from build123d import *

# Parameters (mm, degrees)
F0_W     = 50.8
F0_H     = 31.75
F1_DEPTH = 31.75
F2_W     = 25.4
F2_H     = 19.05
F3_DEPTH = 31.751
F4_R     = 25.4
F5_DEPTH = 50.801


with BuildPart() as f1:
    # F0 (on Front) → F1 (new body)
    with BuildSketch(Plane.XZ):
        with Locations((25.4, 15.875)):
            Rectangle(F0_W, F0_H)
    extrude(amount=F1_DEPTH)

    # F2 (on face) → F3 (cut, through all)
    with BuildSketch(Plane.XZ.offset(31.75)):
        with Locations((25.4, 22.225)):
            Rectangle(F2_W, F2_H)
    extrude(amount=-F3_DEPTH, mode=Mode.SUBTRACT)

    # F4 (on face) → F5 (cut, through all)
    with BuildSketch(Plane.YZ.offset(50.8)):
        with Locations((-31.75, 31.75)):
            Circle(F4_R)
    extrude(amount=-F5_DEPTH, mode=Mode.SUBTRACT)


solid = f1.part
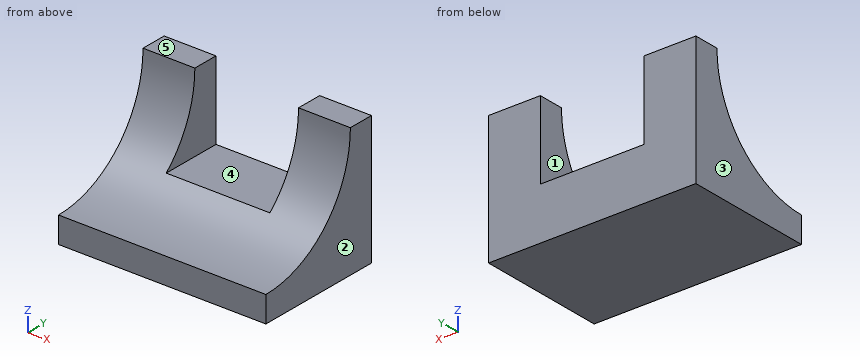
Build history of the part. All positions in model axes, mm. Face numbers are marked on the shaded views. A direction names the side the tool comes from. Round coordinates to 2 decimals unless told otherwise and drop trailing zeros. Loops run counter-clockwise (first coordinate to the right, second up) from the corner with the lowest first, then second, coordinate; pieces in that order, holes last. Notation, with made-up numbers: (51.5, 41.5) -> (91.5, 41.5) arc R27 cw to (91.5, 57.5) -> close; hole circle Ø7 at (33.25, 57.25). An arc over 180 degrees is marked (long way). Use CSV: the item, a comma, the result in double quotes. Start each with the question number.
Q1. Saw through at D-D on z = 22. Give the cut face in (x, y), and give its area (3 significant figures).
Q2. Flat gauge pins, fed straight in: pin 1 Ø7.5 at (x, y) = (27, -7.5) entering from +Z; pin 2 Ø10 at (x, y) = (25.5, -21) entering from +Z; pin 3 Ø1 at (x, y) = (11, -14) entering from +Z. Where does each tip first touch, or does it go through?
Q3. Saw through at A-A on z = 28. Give the cut face in (x, y), and give its area (3 significant figures).
Q4. Mould opens along X. For the marked faces 3, 4 and 5 say: +X half, -X half, draft (parallel to the pull), parting line (faces both ways), or undercut.
Q5. Saw through at C-C on x = 17.5. Give the cut face in (y, z), and give its area (3 significant figures).
Q6. Drill centre lines: L1, parallel to X at y = -8, z = 13; L2, parallel to Z at x = 31.5, y = -12.5; L3, parallel to Z at x = 48, y = -21.5. Where is each one in solid material? Low to high.
Q7. Saw through at B-B on y = -4.5. Give the cut face in (x, z), and give its area (3 significant figures).
Q8. Which spindle directions (+Z, -Z, +X, -X, +Y, -Y) get a long thin tool onto all of the face, cutting with end or side? Do the marked faces 1 and 2. Say none if no direction does.
Solutions:
1,outline,"(0, -8.3) -> (12.7, -8.3) -> (12.7, 0) -> (0, 0) -> close; (38.1, -8.3) -> (50.8, -8.3) -> (50.8, 0) -> (38.1, 0) -> close"
1,area,"211 mm^2"
2,pin 1,"stops at z = 12.7"
2,pin 2,"stops at z = 11.82"
2,pin 3,"stops at z = 14.08"
3,outline,"(0, -6.63) -> (12.7, -6.63) -> (12.7, 0) -> (0, 0) -> close; (38.1, -6.63) -> (50.8, -6.63) -> (50.8, 0) -> (38.1, 0) -> close"
3,area,"168 mm^2"
4,face 3,"-X half"
4,face 4,"undercut"
4,face 5,"draft"
5,outline,"(-31.75, 0) -> (0, 0) -> (0, 12.7) -> (-14.95, 12.7) arc R25.4 cw to (-31.75, 6.35) -> close"
5,area,"330 mm^2"
6,L1,"x = 0 to 12.7, 38.1 to 50.8"
6,L2,"z = 0 to 12.7"
6,L3,"z = 0 to 8.51"
7,outline,"(0, 0) -> (50.8, 0) -> (50.8, 31.75) -> (38.1, 31.75) -> (38.1, 12.7) -> (12.7, 12.7) -> (12.7, 31.75) -> (0, 31.75) -> close"
7,area,"1,130 mm^2"
8,face 1,"+Z, +Y, -Y"
8,face 2,"+Z, -Z, +X, +Y, -Y"
